Geometry: final body of the model. Coordinates: model frame, mm. A direction names the side the tool comes from. Round coordinates to 2 decimals unless told otherwise and drop trailing zeros. Write each loop counter-clockwise with the first axis right and the second up, starting at its lowest first coordinate (ties: lowest second). Pieces come first, ordered by that corner, then holes. Notation, with made-up numbers: (-14.75, -22) - (43.25, -22) arc R20 ccw to (43.25, 16) - close; hole circle Ø10 at (-14.5, 87). An arc over 180 degrees is marked (long way). Write each question's results on one line, items separated by ' | '.
Autodesk Fusion 360 part; units mm, degrees
sketch "Boceto1" plane through (0, 0, 0) normal (0, 1, 0) x (1, 0, 0)
  line L0 (-50, 50) -> (-50, -10)
  line L1 (-50, 50) -> (-15, 50)
  line L2 (-15, 50) -> (-15, -10)
  line L3 (-15, -10) -> (-50, -10)
  dimension "d1" = 60
  dimension "d2" = 35
extrude "Extruir1" add sketch "Boceto1" along normal blind 3
sketch "Boceto2" plane through (0, 0, 0) normal (0, -1, 0) x (1, 0, 0)
  line L0 (-50, 10) -> (-50, -50)
  line L1 (-50, -50) -> (-15, -50)
  line L2 (-15, -50) -> (-15, 10)
  line L3 (-15, 10) -> (-50, 10)
  line L4 (-35.5, -40) -> (-34.4961, -23.8757)
  line L5 (-29.5, -40) -> (-30.5039, -23.8757)
  arc A0 (-30.5039, -23.8757) -> (-34.4961, -23.8757) centre (-32.5, -24) ccw
  arc A1 (-35.5, -40) -> (-29.5, -40) centre (-32.5, -40) ccw
  arc A2 (-35.5, -40) -> (-29.5, -40) centre (-32.5, -40) ccw
extrude "Extruir2" add 1 faces at (-38.3333, 3, -30) along direction (0, 1, 0) blind 2
extrude "Extruir3" cut sketch "Boceto2" against normal blind 2 contours L4 L5 A0 A1 A2
sketch "Boceto3" plane through (0, 5, 0) normal (0, 1, 0) x (-1, 0, 0)
  line L0 (50, -50) -> (50, 10)
  line L1 (50, 10) -> (15, 10)
  line L2 (15, 10) -> (15, -50)
  line L3 (15, -50) -> (50, -50)
  line L4 (39, -12) -> (39, 2)
  line L5 (39, 2) -> (37, 2)
  line L6 (37, 2) -> (37, -12)
  line L7 (50, 10) -> (32.5, 10)
  line L8 (32.5, -9) -> (37, -12)
  line L9 (28, 2) -> (26, 2)
  line L10 (26, 2) -> (26, -12)
  line L11 (28, 2) -> (28, -12)
  line L12 (28, -12) -> (32.5, -9)
  line L13 (39, -12) -> (39, -14)
  line L14 (39, -14) -> (37, -14)
  line L15 (37, -14) -> (32.5, -11)
  line L16 (32.5, -11) -> (28, -14)
  line L17 (28, -14) -> (26, -14)
  line L18 (26, -14) -> (26, -12)
extrude "Extruir4" cut sketch "Boceto3" against normal blind 2 contours L4 L5 L6 L8 L9 L10 L11 L12 L13 L14 L15 L16 L17 L18
Q1. Access query for faces 1 (the cylindrical face through (-32.5, 1, -22)), 2 (the flat face through (-33, 0, -20)), 3 (the flat face through (-39, 4, -6)). Directions: +Z, -Z, +X, -X, +Y, -Y. A direction counts if a zero-diameter tool reaches every point of the face in a straight line with its end or side. Return the directions, or none.
Answer block:
face 1: -Y | face 2: +Z, -Z, +X, -X, -Y | face 3: +Y
Q2. Mould query, pull axis X, two halves, no side actions, for faces 4 (the flat face through (-15, 2, -20)), 5 (the flat face through (-50, 2, -20)), 6 (the flat face through (-35, 1, -32)), 7 (the flat face through (-37, 4, -5)). Classes: pulls with the +X half, pulls with the -X half, needs draft (parallel to the pull), parting line crosses it, or undercut.
Answer block:
face 4: pulls with the +X half | face 5: pulls with the -X half | face 6: undercut | face 7: undercut
Q3. Section query A-A, the plane z = -38.5. Return loops of the section in (x, y).
Answer block:
outline: (-50, 0) - (-35.41, 0) - (-35.41, 2) - (-29.59, 2) - (-29.59, 0) - (-15, 0) - (-15, 5) - (-50, 5) - close
Q4. Ray query, line 1 along X through (y, z) = (4.2, -10.5); line 2 along Y through (x, z) = (-30.5, -25); line 3 along X through (y, z) = (0.6, -37). Return the intervals inside material, ascending.
Answer block:
line 1: -50 to -39, -37 to -34.75, -30.25 to -28, -26 to -15 | line 2: 2 to 5 | line 3: -50 to -35.31, -29.69 to -15
